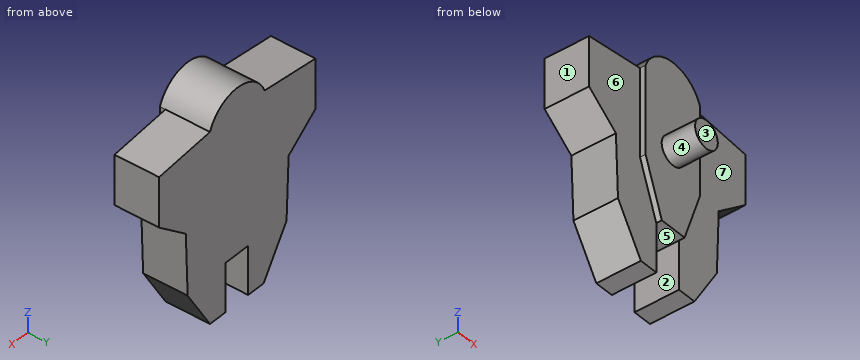
from build123d import *

# Parameters (mm, degrees)
BOSS_EXTRUDE1_DEPTH = 9
SKETCH3_R           = 2.5
BOSS_EXTRUDE2_DEPTH = 6
CUT_EXTRUDE1_DEPTH  = 1


with BuildPart() as part:
    # Sketch2 → Boss-Extrude1 (new body)
    with BuildSketch(Plane(origin=(0, 0, 0), x_dir=(1, 0, 0), z_dir=(0, 1, 0))):
        with BuildLine():
            Line((21.423631539, 59.756571467), (21.423631539, 67.28012571))
            Line((21.423631539, 67.28012571), (27.320471351, 71.956929699))
            Line((27.320471351, 71.956929699), (27.777984785, 83.191426238))
            Line((27.777984785, 83.191426238), (32.810632556, 91.223328742))
            Line((32.810632556, 91.223328742), (36.210632556, 91.223328742))
            Line((36.210632556, 91.223328742), (36.210632556, 82.473328742))
            Line((36.210632556, 82.473328742), (41.210632556, 82.473328742))
            Line((41.210632556, 82.473328742), (41.210632556, 91.223328742))
            Line((41.210632556, 91.223328742), (44.610632556, 91.223328742))
            Line((44.610632556, 91.223328742), (49.541610675, 83.191426238))
            Line((49.541610675, 83.191426238), (49.948289283, 71.956929699))
            Line((49.948289283, 71.956929699), (55.823631539, 67.28012571))
            Line((55.823631539, 67.28012571), (55.823631539, 58.333196339))
            Line((55.823631539, 58.333196339), (44.623631539, 57.163995342))
            ThreePointArc((44.623631539, 57.163995342), (38.623631539, 53.004094152), (32.623631539, 57.163995342))
            Line((32.623631539, 57.163995342), (21.423631539, 58.333196339))
            Line((21.423631539, 58.333196339), (21.423631539, 59.756571467))
        make_face()
    extrude(amount=BOSS_EXTRUDE1_DEPTH)

    # Sketch3 → Boss-Extrude2 (add)
    with BuildSketch(Plane.XZ):
        with Locations((38.670089984, -68.740632333)):
            Circle(SKETCH3_R)
    extrude(amount=BOSS_EXTRUDE2_DEPTH)

    # Sketch4 → Cut-Extrude1 (cut)
    with BuildSketch(Plane.XZ):
        Polygon((32.623631539, -57.163995342), (21.423631539, -58.333196339), (21.423631539, -67.28012571), (27.320471351, -71.956929699), (27.777984785, -83.191426238), (32.810632556, -91.223328742), (36.210632556, -91.223328742), (36.210632556, -82.473328742), (32.623631539, -72.967523608), align=None)
        Polygon((44.623631539, -57.163995342), (44.623631539, -72.967523608), (41.210632556, -82.473328742), (41.210632556, -91.223328742), (44.610632556, -91.223328742), (49.541610675, -83.191426238), (49.948289283, -71.956929699), (55.823631539, -67.28012571), (55.823631539, -58.333196339), align=None)
    extrude(amount=-CUT_EXTRUDE1_DEPTH, mode=Mode.SUBTRACT)


solid = part.part
The listing builds one solid part. Answer for the finished solid, in the listing's coordinates (mm). Face numbers are marked on the shaded views. A direction names the side the tool comes from. Coordinates: 2 decimals unless noted, no trailing zeros. Order: outer loops, then holes, each group sorted by start corner. A loop starts at its lowest first (then second) coordinate and runs counter-clockwise, first axis right, second up.
Q1. A cutting plane is placed at C-C, the plane x = 40.5. Write down the section's boundary in (y, z), and give its area (3 significant figures).
Q2. Given P1, Ø2.5, axis at y = 3.5, z = -85, coming from the +X side; P2, Ø10, axis at x = 50.5, z = -85.5, coming from the -Y side; P3, Ø0.8, axis at y = 0.5, z = -65, coming from the +X side, each flat-ended and moving along its own axis, determine where each tip first touches the part or whether it passes through.
Q3. Consider line 1 (X direction, y = 3.5, z = -83); line 2 (Y direction, x = 39, z = -60); line 3 (Y direction, x = 24.5, z = -65). Determine where each line is inside the solid, lowest interval first.
Q4. A cutting plane is placed at B-B, the plane z = -60. Write down the section's boundary in (x, y).
Q5. A cutting plane is placed at A-A, the plane y = 5. Write down the section's boundary in (x, z).
Q6. Which of the six approach directions +Z, -Z, +X, -X, +Y, -Y give full straight-line access (tool end or side, diameter ignored) to the marked faces 4, 5, 6 and 7?
Q7. A cutting plane is placed at D-D, the plane x = 34. Write down the section's boundary in (y, z) (3 decimals).
Q8. For a pull along X with two mould halves and no side action, classify the marked faces 1, 2 and 3 as pulls with the +X half, pulls with the -X half, needs draft (parallel to the pull), parting line crosses it, or undercut.
Answers follow:
1. outline: (-6, -70.44) - (0, -70.44) - (0, -82.47) - (9, -82.47) - (9, -53.29) - (0, -53.29) - (0, -67.04) - (-6, -67.04) - close
1. area: 283 mm2
2. P1: stops at x = 49.2
2. P2: stops at y = 1
2. P3: stops at x = 44.62
3. line 1: x = 27.77 to 36.21, 41.21 to 49.55
3. line 2: y = 0 to 9
3. line 3: y = 1 to 9
4. outline: (21.42, 1) - (32.62, 1) - (32.62, 0) - (44.62, 0) - (44.62, 1) - (55.82, 1) - (55.82, 9) - (21.42, 9) - close
5. outline: (21.42, -67.28) - (27.32, -71.96) - (27.78, -83.19) - (32.81, -91.22) - (36.21, -91.22) - (36.21, -82.47) - (41.21, -82.47) - (41.21, -91.22) - (44.61, -91.22) - (49.54, -83.19) - (49.95, -71.96) - (55.82, -67.28) - (55.82, -58.33) - (44.62, -57.16) arc R6.41 ccw to (32.62, -57.16) - (21.42, -58.33) - close
6. face 4: -Y
6. face 5: -Z, +Y, -Y
6. face 6: -Z, -X, -Y
6. face 7: -Z, +X, -Y
7. outline: (0, -76.615) - (1, -76.615) - (1, -91.223) - (9, -91.223) - (9, -54.976) - (0, -54.976) - close
8. face 1: pulls with the -X half
8. face 2: undercut
8. face 3: needs draft
